Autodesk Inventor part; units mm, degrees
ref_plane "YZ Plane" through (0, 0, 0) normal (1, 0, 0) x (0, 1, 0)
ref_plane "XZ Plane" through (0, 0, 0) normal (0, 1, 0) x (-1, 0, 0)
ref_plane "XY Plane" through (0, 0, 0) normal (0, 0, 1) x (1, 0, 0)
sketch "Sketch1" plane through (0, 0, 0) normal (1, 0, 0) x (0, 1, 0)
  line L0 (-50, -71) -> (50, -71)
  line L1 (50, -71) -> (50, 71)
  line L2 (50, 71) -> (-50, 71)
  line L3 (-50, 71) -> (-50, -71)
  line L4 (-50, -71) -> (50, 71) construction
  line L5 (50, -71) -> (-50, 71) construction
  point P0 (0, 0)
  dimension "d0" = 100
  dimension "d1" = 142
extrude "Extrusion1" add sketch "Sketch1" along normal blind 3
sketch "Sketch2" plane through (3, 0, 0) normal (1, 0, 0) x (0, 0, -1)
  line L0 (-71, -50) -> (71, -50)
  line L1 (-5, -50) -> (-25, -50)
  line L2 (-25, -50) -> (-25, -53)
  line L3 (-25, -53) -> (-5, -53)
  line L4 (-5, -53) -> (-5, -50)
  line L5 (-45, -50) -> (-65, -50)
  line L6 (-65, -50) -> (-65, -53)
  line L7 (-65, -53) -> (-45, -53)
  line L8 (-45, -53) -> (-45, -50)
  point P0 (0, 0)
  dimension "d4" = 20
  dimension "d5" = 3
  dimension "d6" = 5
  dimension "d7" = 20
  dimension "d8" = 3
  dimension "d9" = 20
extrude "Extrusion2" add sketch "Sketch2" against normal blind 4
mirror "Mirror1" about plane through (0, 0, 0) normal (0, 0, 1) of "Extrusion2"
sketch "Sketch3" plane through (3, 0, 0) normal (1, 0, 0) x (0, 0, -1)
  line L0 (-60, -30) -> (-57, -30)
  line L1 (-57, -30) -> (-57, -45)
  line L2 (-57, -45) -> (-60, -45)
  line L3 (-60, -45) -> (-60, -30)
  line L4 (-71, -50) -> (-65, -50)
  point P0 (0, 0)
  dimension "d12" = 3
  dimension "d13" = 15
  dimension "d14" = 57
  dimension "d15" = 5
extrude "Extrusion3" cut sketch "Sketch3" against normal blind 4
properties part number "frount plate"
Input: part model. Units: mm. Frame: model coordinates. A direction names the side the tool comes from. Coordinates: 2 decimals unless noted, no trailing zeros. Write each loop counter-clockwise with the first axis right and the second up, starting at its lowest first coordinate (ties: lowest second). Pieces come first, ordered by that corner, then holes.
1) Material intervals for line 1 along Z through (x, y) = (0.75, -31); line 2 along X through (y, z) = (-2, -13.5); line 3 along Y through (x, z) = (1.4, -39.5), sorted ascending.
2) Set-up query: faces 1 (the flat face through (1, -52, -25)), 2 (the flat face through (1, -50, 68)), 3 (the flat face through (2, -45, 58)). Return all of +Z, -Z, +X, -X, +Y, -Y with unobstructed straight access to the full face (end or side cutting, diameter ignored); none if empty.
3) Section C-C on z = 16.5. Output: boundary loops of the cut face in (x, y), and give its area (3 significant figures).
4) Section D-D on y = 40. Output: boundary loops of the cut face in (x, z).
5) Pin query (flat end, axial travel): pin 1 Ø0.9 at (x, z) = (1, 69.5) entering from -Y; pin 2 Ø3 at (y, z) = (21.5, 43) entering from -X; pin 3 Ø1.5 at (x, y) = (1.5, -51) entering from -Z. Return the tip coordinate at first contact, or that it passes through.
6) Section B-B on x = 1.85. Output: boundary loops of the cut face in (y, z), and give its area (3 significant figures).
7) Section A-A on y = -40. Output: boundary loops of the cut face in (x, z), and give its area (3 significant figures).
Check result:
1. line 1: z = -71 to 57, 60 to 71
1. line 2: x = 0 to 3
1. line 3: y = -50 to 50
2. face 1: +X, -X, -Y
2. face 2: +Z, +X, -X, -Y
2. face 3: +X, -X
3. outline: (-1, -53) - (3, -53) - (3, 50) - (0, 50) - (0, -50) - (-1, -50) - close
3. area: 312 mm2
4. outline: (0, -71) - (3, -71) - (3, 71) - (0, 71) - close
5. pin 1: stops at y = -50
5. pin 2: stops at x = 0
5. pin 3: stops at z = -65
6. outline: (-53, -65) - (-50, -65) - (-50, -71) - (50, -71) - (50, 71) - (-50, 71) - (-50, 65) - (-53, 65) - (-53, 45) - (-50, 45) - (-50, 25) - (-53, 25) - (-53, 5) - (-50, 5) - (-50, -5) - (-53, -5) - (-53, -25) - (-50, -25) - (-50, -45) - (-53, -45) - close; hole (-45, 57) - (-30, 57) - (-30, 60) - (-45, 60) - close
6. area: 14,400 mm2
7. outline: (0, -71) - (3, -71) - (3, 57) - (0, 57) - close; (0, 60) - (3, 60) - (3, 71) - (0, 71) - close
7. area: 417 mm2
